```python
from build123d import *

# Parameters (mm, degrees)
F0_W     = 61.6851523519
F0_H     = 115.4553033412
F1_DEPTH = 112.395
F2_DEPTH = 224.79
F3_W     = 91.9657982886
F3_H     = 36.7413535714
F3_W_2   = 27.7609527111
F3_H_2   = 13.8463228941
F3_W_3   = 20.4830765724
F3_H_3   = 32.7579472214
F4_DEPTH = 65.405


with BuildPart() as f1:
    # F0 (on Top) → F1 (new body)
    with BuildSketch(Plane.XY):
        with Locations((-30.8425761759, -0.1723002642)):
            Rectangle(F0_W, F0_H)
    extrude(amount=F1_DEPTH)

    # F2 (add): a face of the model
    f2_faces = [f1.faces().sort_by_distance(p)[0] for p in [
        (0, -0.1723002642, 56.1975),
    ]]
    extrude(f2_faces, amount=F2_DEPTH)

    # F3 (on face) → F4 (cut)
    with BuildSketch(Plane.XZ.offset(57.8999519348)):
        with Locations((88.7409579009, 74.1017498076)):
            Rectangle(F3_W, F3_H)
        with Locations((96.7281907797, 75.1979798079)):
            Rectangle(F3_W_2, F3_H_2, mode=Mode.SUBTRACT)
        with Locations((165.1449352503, 39.1824124381)):
            Rectangle(F3_W_3, F3_H_3)
    extrude(amount=-F4_DEPTH, mode=Mode.SUBTRACT)


solid = f1.part
```
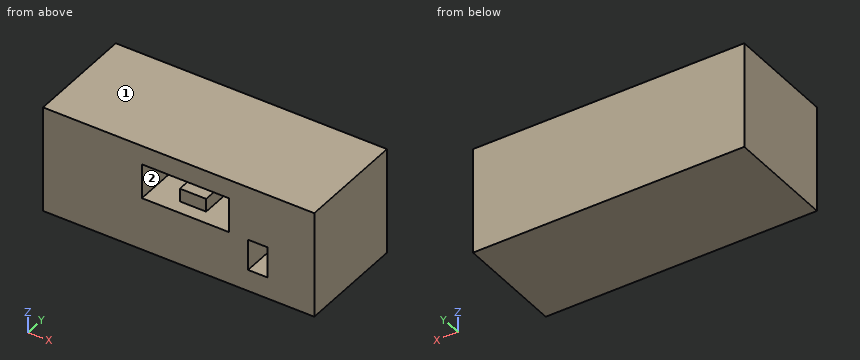
For this review, take the finished solid that the model builds, in its own axes (mm). Face numbers are marked on the shaded views. A direction names the side the tool comes from. Coordinates: 2 decimals unless noted, no trailing zeros. Write each loop counter-clockwise with the first axis right and the second up, starting at its lowest first coordinate (ties: lowest second). Pieces come first, ordered by that corner, then holes.
(1) Tool access review of the marked faces 1 and 2: name each direction out of +Z, -Z, +X, -X, +Y, -Y from which nothing blocks a thin tool from reaching the whole face with its end or side.
(2) Add section A-A on y = -39.5. Give the boundary of the cut face in (x, z) (3 decimals), then the cut area to 3 significant figures.
(3) Add section C-C on x = 69. Give the boundary of the cut face in (y, z) (3 decimals).
(4) Wall thickness on probe 1 along X at (y, z) = (-48.5, 76.5); probe 2 along X at (y, z) = (-2.5, 53); probe 3 along X at (y, z) = (-52.5, 60.5): over which ranges is each line inside the solid? List them lowest first.
(5) Add section B-B on z = 75. Give the boundary of the cut face in (x, y), then the cut area to 3 significant figures.
Answer sheet:
1. face 1: +Z, +X, -X, +Y, -Y
1. face 2: -Y
2. outline: (-61.685, 0) - (224.79, 0) - (224.79, 112.395) - (-61.685, 112.395) - close; (82.848, 68.275) - (110.609, 68.275) - (110.609, 82.121) - (82.848, 82.121) - close; hole (42.758, 55.731) - (134.724, 55.731) - (134.724, 92.472) - (42.758, 92.472) - close; hole (154.903, 22.803) - (175.386, 22.803) - (175.386, 55.561) - (154.903, 55.561) - close
2. area: 28,500 mm2
3. outline: (-57.9, 0) - (57.555, 0) - (57.555, 112.395) - (-57.9, 112.395) - (-57.9, 92.472) - (7.505, 92.472) - (7.505, 55.731) - (-57.9, 55.731) - close
4. probe 1: x = -61.69 to 42.76, 82.85 to 110.61, 134.72 to 224.79
4. probe 2: x = -61.69 to 154.9, 175.39 to 224.79
4. probe 3: x = -61.69 to 42.76, 134.72 to 224.79
5. outline: (-61.69, -57.9) - (42.76, -57.9) - (42.76, 7.51) - (82.85, 7.51) - (82.85, -57.9) - (110.61, -57.9) - (110.61, 7.51) - (134.72, 7.51) - (134.72, -57.9) - (224.79, -57.9) - (224.79, 57.56) - (-61.69, 57.56) - close
5. area: 28,900 mm2
